Study the drawing (mm; zero at the part's minimum x, y, z) and answer. Coordinates: 2 decimals unless noted, no trailing zeros. Loops run counter-clockwise (first coordinate to the right, second up) from the corner with the lowest first, then second, coordinate; pieces in that order, holes last. Notation, with made-up numbers: (38.25, 3) - (79.25, 3) arc R18 ccw to (79.25, 35) - close; hole circle Ø2 at (20, -17). An arc over 180 degrees is marked (long way). Put each result on its own line as item: value.
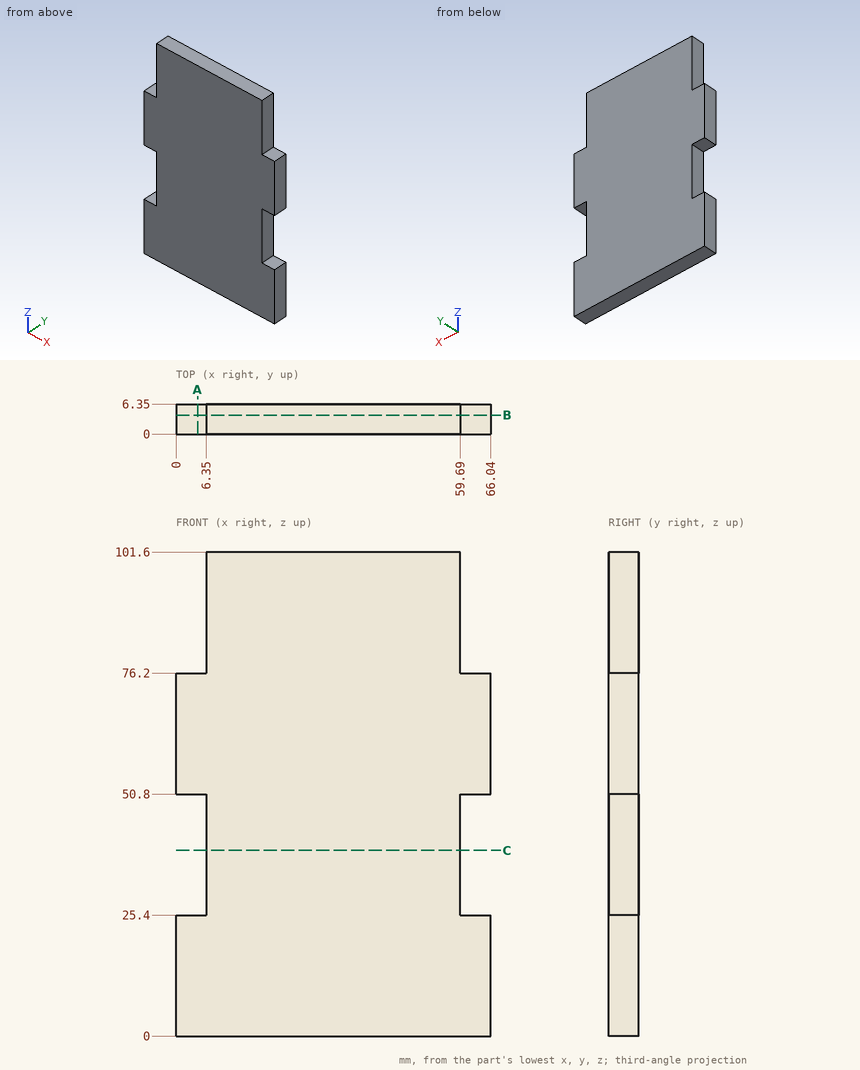
1) The part is cut by section B-B (y = 4). Give the vertices of the cut face in (x, z).
Found:
outline: (0, 0) - (66.04, 0) - (66.04, 25.4) - (59.69, 25.4) - (59.69, 50.8) - (66.04, 50.8) - (66.04, 76.2) - (59.69, 76.2) - (59.69, 101.6) - (6.35, 101.6) - (6.35, 76.2) - (0, 76.2) - (0, 50.8) - (6.35, 50.8) - (6.35, 25.4) - (0, 25.4) - close
2) Straight lines are drawn through the part: L1, parallel to Z at x = 3, y = 4.5; L2, parallel to X at y = 5.25, z = 95.5. For each, find the intervals that lie inside material, in ascending order. Write a range as [from, to].
Found:
L1: z = [0, 25.4], [50.8, 76.2]
L2: x = [6.35, 59.69]
3) The part is cut by section C-C (z = 39). Give the vertices of the cut face in (x, y).
Found:
outline: (6.35, 0) - (59.69, 0) - (59.69, 6.35) - (6.35, 6.35) - close
4) The part is cut by section A-A (x = 4.5). Give the vertices of the cut face in (y, z).
Found:
outline: (0, 0) - (6.35, 0) - (6.35, 25.4) - (0, 25.4) - close; (0, 50.8) - (6.35, 50.8) - (6.35, 76.2) - (0, 76.2) - close
5) Each of these flat-tipped pins is pushed along its axis until it touches: pin 1 (3 mm diameter, centred on y = 4, z = 42.5, fed in from +X); pin 2 (1.9 mm diameter, centred on y = 2.5, z = 42.5, fed in from -X); pin 3 (3 mm diameter, centred on x = 61.5, y = 2.5, fed in from +Z). Where does it stop, or does it pass through?
Found:
pin 1: stops at x = 59.69
pin 2: stops at x = 6.35
pin 3: stops at z = 76.2
